Verification items for the finished model (mm, model axes). Coordinates: 2 decimals unless noted, no trailing zeros. Write each loop counter-clockwise with the first axis right and the second up, starting at its lowest first coordinate (ties: lowest second). Pieces come first, ordered by that corner, then holes. Notation, with made-up numbers: (13, 37) - (29, 37) arc R25 cw to (29, 63) - close; hole circle Ø5 at (79.25, 69). An arc over 180 degrees is marked (long way). Use one line per item in the form item = value. Start each with the question number.
(1) Sectioned sample at B-B (x = 87.5). Record the cut outline in (y, z), and give its area (3 significant figures).
(2) Sectioned sample at C-C (z = 1.4). Record the cut outline in (x, y) (3 decimals).
(3) Gauge pin test, flat ends, axial feed: pin 1 Ø6 at (x, y) = (25.5, 32.5) entering from +Z; pin 2 Ø2 at (y, z) = (-53.5, 2) entering from -X; pin 3 Ø3 at (x, z) = (-61.5, 1.5) entering from -Y. Record the tip position at first contact, or that the pin passes through.
(4) Sectioned sample at A-A (x = 0). Record the cut outline in (y, z) (3 decimals), and give its area (3 significant figures).
(5) Sectioned sample at D-D (y = -87.5). Record the cut outline in (x, z).
(6) Material ranges on line 1 (Y direction, x = 0, z = 1.6) (3 decimals); line 2 (Y direction, x = -2.5, z = 0.6); line 3 (X direction, y = 23.5, z = 3.8), recorded low to high. Write a range as [from, to].
from build123d import *

# Parameters (mm, degrees)
F0_R     = 97.79
F0_R_2   = 5
F0_R_3   = 45.085
F1_DEPTH = 5
F3_DEPTH = 5.001


# Not quite as in the source:
# - a feature names something its author has since deleted; it is built from what else it names


with BuildPart() as f1:
    # F0 (on Top) → F1 (new body)
    with BuildSketch(Plane.XY):
        Circle(F0_R)
        with Locations((0, -87.5)):
            Circle(F0_R_2, mode=Mode.SUBTRACT)
        with Locations((-87.5, 0)):
            Circle(F0_R_2, mode=Mode.SUBTRACT)
        Circle(F0_R_3, mode=Mode.SUBTRACT)
        with Locations((87.5, 0)):
            Circle(F0_R_2, mode=Mode.SUBTRACT)
        with Locations((0, 87.5)):
            Circle(F0_R_2, mode=Mode.SUBTRACT)
    extrude(amount=F1_DEPTH)

    # F2 (on face) → F3 (cut, through all)
    with BuildSketch(Plane.XY.offset(5)):
        with BuildLine():
            ThreePointArc((97.4057710678, 8.6602461102), (69.1479721322, 69.1479721322), (8.6602461102, 97.4057710678))
            Line((8.6602461102, 97.4057710678), (97.4057710678, 8.6602461102))
        make_face()
    extrude(amount=-F3_DEPTH, mode=Mode.SUBTRACT)


solid = f1.part
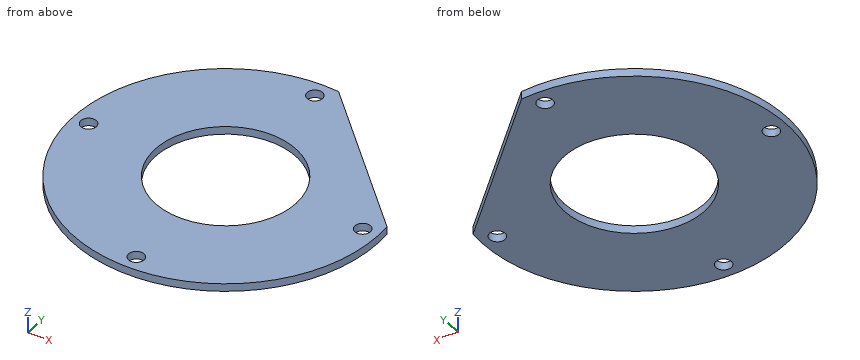
Answers below:
q1.outline = (-43.67, 0) - (-5, 0) - (-5, 5) - (-43.67, 5) - close; (5, 0) - (18.57, 0) - (18.57, 5) - (5, 5) - close
q1.area = 261 mm2
q2.outline = (8.66, 97.406) arc R97.79 ccw (long way) to (97.406, 8.66) - close; hole circle Ø10 at (-87.5, 0); hole circle Ø90.17 at (0, 0); hole circle Ø10 at (0, -87.5); hole circle Ø10 at (0, 87.5); hole circle Ø10 at (87.5, 0)
q3.pin_1 = through
q3.pin_2 = -82.5
q3.pin_3 = -77.22
q4.outline = (-97.79, 0) - (-92.5, 0) - (-92.5, 5) - (-97.79, 5) - close; (-82.5, 0) - (-45.085, 0) - (-45.085, 5) - (-82.5, 5) - close; (45.085, 0) - (82.5, 0) - (82.5, 5) - (45.085, 5) - close; (92.5, 0) - (97.79, 0) - (97.79, 5) - (92.5, 5) - close
q4.area = 427 mm2
q5.outline = (-43.67, 0) - (-5, 0) - (-5, 5) - (-43.67, 5) - close; (5, 0) - (43.67, 0) - (43.67, 5) - (5, 5) - close
q6.line_1 = [-97.79, -92.5], [-82.5, -45.085], [45.085, 82.5], [92.5, 97.79]
q6.line_2 = [-97.76, -91.83], [-83.17, -45.02], [45.02, 83.17], [91.83, 97.76]
q6.line_3 = [-94.92, -38.48], [38.48, 82.57]
